Part model, mm, in its own coordinate system. Face numbers are marked on the shaded views. A direction names the side the tool comes from. Coordinates: 2 decimals unless noted, no trailing zeros. Loops run counter-clockwise (first coordinate to the right, second up) from the corner with the lowest first, then second, coordinate; pieces in that order, holes last.
```python
from build123d import *

# Parameters (mm, degrees)
SKETCH_2_R          = 2.95
SKETCH_2_R_2        = 1.55
EXTRUDE_1_DEPTH     = 20
SKETCH_3_W          = 53.999961589
SKETCH_3_H          = 13.8
CUT_EXTRUDE_1_DEPTH = 10
SKETCH_4_R          = 21.1
CUT_EXTRUDE_2_DEPTH = 7
SKETCH_5_R          = 19
CUT_EXTRUDE_3_DEPTH = 0.8
CHAMFER_1_SIZE      = 1
SKETCH_6_R          = 3
CUT_EXTRUDE_4_DEPTH = 3


with BuildPart() as part:
    # 草图2 → 凸台-拉伸1 (new body)
    with BuildSketch(Plane.XY):
        with BuildLine():
            Line((-24.99119492, 0.663496162), (-27, -90))
            Line((-27, -90), (0, -90))
            Line((0, -90), (26.999961589, -90))
            Line((26.999961589, -90), (24.991195257, 0.663483484))
            ThreePointArc((24.991195257, 0.663483484), (6.341e-06, 25.000001014), (-24.99119492, 0.663496162))
        make_face()
        Circle(SKETCH_2_R, mode=Mode.SUBTRACT)
        with Locations((-15, -83)):
            Circle(SKETCH_2_R_2, mode=Mode.SUBTRACT)
        with Locations((0, -83)):
            Circle(SKETCH_2_R_2, mode=Mode.SUBTRACT)
        with Locations((15, -83)):
            Circle(SKETCH_2_R_2, mode=Mode.SUBTRACT)
    extrude(amount=EXTRUDE_1_DEPTH)

    # 草图3 → 切除-拉伸1 (cut)
    with BuildSketch(Plane.XY.offset(20)):
        with Locations((-1.9205e-05, -83.1)):
            Rectangle(SKETCH_3_W, SKETCH_3_H)
    extrude(amount=-CUT_EXTRUDE_1_DEPTH, mode=Mode.SUBTRACT)

    # 草图4 → 切除-拉伸2 (cut)
    with BuildSketch(Plane.XY.offset(20)):
        Circle(SKETCH_4_R)
    extrude(amount=-CUT_EXTRUDE_2_DEPTH, mode=Mode.SUBTRACT)

    # 草图5 → 切除-拉伸3 (cut)
    with BuildSketch(Plane.XY.offset(13)):
        Circle(SKETCH_5_R)
    extrude(amount=-CUT_EXTRUDE_3_DEPTH, mode=Mode.SUBTRACT)

    # 倒角1
    chamfer_1_edges = [part.edges().sort_by_distance(p)[0] for p in [
        (25.84270003, -37.768258258, 20),
        (6.341e-06, 25.000001014, 20),
        (25.995578423, -44.668258258, 0),
        (-21.1, 0, 20),
        (-25.99559746, -44.668251919, 0),
        (6.341e-06, 25.000001014, 0),
        (-25.842716139, -37.768251919, 20),
    ]]
    chamfer(chamfer_1_edges, length=CHAMFER_1_SIZE)

    # 草图6 → 切除-拉伸4 (cut)
    with BuildSketch(Plane(origin=(0, 0, 0), x_dir=(-1, 0, 0), z_dir=(0, 0, -1))):
        with Locations((-15, -83)):
            Circle(SKETCH_6_R)
        with Locations((0, -83)):
            Circle(SKETCH_6_R)
        with Locations((15, -83)):
            Circle(SKETCH_6_R)
    extrude(amount=-CUT_EXTRUDE_4_DEPTH, mode=Mode.SUBTRACT)


solid = part.part
```
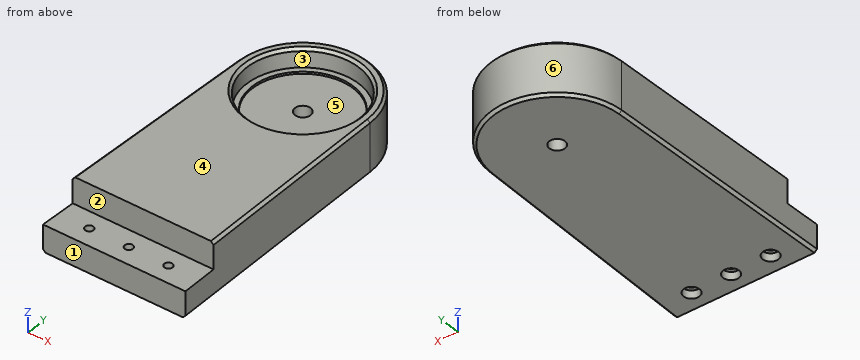
Q1. Drop flat-ended pins along their axis: P1, Ø5.5, axis at x = -15, y = -83, coming from the +Z side; P2, Ø5, axis at x = 0, y = -83, coming from the -Z side; P3, Ø4, axis at y = -15.5, z = 7, coming from the +X side; P4, Ø4, axis at x = -4.5, y = -77, coming from the +Z side. Give the stop position or say it passes through.
Q2. Probe line 1 (Y direction, x = -15, z = 3.25); line 2 (Y direction, x = 0, z = 12); line 3 (Z direction, x = -7.5, y = -15). List the from-to ranges inside material, lowest first.
Q3. Saw through at A-A (x = 0). Count the separate pieces of the cut face and the enclosed holes in it, plus the area to 3 significant figures.
Q4. Tool access for the marked faces 1 and 2: list every direction of +Z, -Z, +X, -X, +Y, -Y with a clear straight run to the whole face (end or side of a thin tool).
Q5. Mould opens along Y. For the marked faces 3, 4, 5 and 6 say: released by +Y, released by -Y, zero draft, split by the parting line, or undercut.
Q6. Saw through at D-D (y = -32.5). List the corners of the cut face in (x, z), plus the area to 3 significant figures.
Q7. Saw through at B-B (z = 8.25). List the corners of the cut face in (x, y).
Checked values:
1. P1: stops at z = 10
1. P2: stops at z = 3
1. P3: stops at x = 25.39
1. P4: stops at z = 20
2. line 1: y = -90 to -84.55, -81.45 to 20
2. line 2: y = -76.2 to -2.95, 2.95 to 25
2. line 3: z = 0 to 12.2
3. separate pieces: 3
3. enclosed holes: 0
3. area: 1,720 mm2
4. face 1: +Z, -Z, +X, -X, -Y
4. face 2: +Z, +X, -X, -Y
5. face 3: undercut
5. face 4: zero draft
5. face 5: undercut
5. face 6: released by +Y
6. outline: (-25.73, 1) - (-24.73, 0) - (24.73, 0) - (25.73, 1) - (25.73, 19) - (24.73, 20) - (-24.73, 20) - (-25.73, 19) - close
6. area: 1,030 mm2
7. outline: (-27, -90) - (27, -90) - (24.99, 0.66) arc R25 ccw to (-24.99, 0.66) - close; hole circle Ø3.1 at (-15, -83); hole circle Ø5.9 at (0, 0); hole circle Ø3.1 at (0, -83); hole circle Ø3.1 at (15, -83)
